Can you work these out from the model? Positions are in its coordinate system, mm. A direction names the side the tool comes from. Round coordinates to 2 decimals unless told otherwise and drop trailing zeros. Loops run counter-clockwise (first coordinate to the right, second up) from the corner with the lowest first, then second, coordinate; pieces in that order, holes last. Notation, with made-up numbers: (-30.75, 80.5) - (-20.75, 80.5) arc R15 cw to (-20.75, 92.5) - close; hole circle Ø2 at (-29, 68). An arc over 180 degrees is marked (long way). Answer as CSV lines item,"result".
```python
from build123d import *

# Parameters (mm, degrees)
F0_W     = 25.4
F0_H     = 5.5252907636
F0_H_2   = 3.9997092364
F0_H_3   = 19.05
F1_DEPTH = 63.5


with BuildPart() as f1:
    # F0 (on Front) → F1 (new body, symmetric)
    with BuildSketch(Plane.XZ):
        with BuildLine():
            ThreePointArc((57.15, 62.6752907636), (56.5270735546, 62.6697350267), (55.9043452947, 62.6530695835))
            add(Edge.make_bspline(
                [(55.9043452947, 62.6530695835), (56.3224009601, 62.6625285107), (56.7376574323, 62.6699360436), (57.15, 62.6752907636)],
                knots=[110.6508010744, 110.6508010744, 110.6508010744, 110.6508010744, 111.8589917407, 111.8589917407, 111.8589917407, 111.8589917407], degree=3))
        make_face()
        with BuildLine():
            add(Edge.make_bspline(
                [(-41.275, 9.525), (-44.1485205161, 43.7142056375), (17.617181224, 61.7867842379), (55.9043452947, 62.6530695835)],
                knots=[0, 0, 0, 0, 110.6508010744, 110.6508010744, 110.6508010744, 110.6508010744], degree=3))
            Line((-41.275, 9.525), (22.225, 9.525))
            Line((22.225, 9.525), (22.225, 27.7502907636))
            ThreePointArc((22.225, 27.7502907636), (32.0177486525, 52.0015910835), (55.9043452947, 62.6530695835))
        make_face()
        with Locations((73.025, 40.8626453818)):
            Rectangle(F0_W, F0_H)
        with Locations((73.025, 64.6751453818)):
            Rectangle(F0_W, F0_H_2)
        Polygon((85.725, 66.675), (85.725, 62.6752907636), (85.725, 43.6252907636), (85.725, 38.1), (111.125, 38.1), (111.125, 66.675), align=None)
        with BuildLine():
            Line((22.225, 27.7502907636), (22.225, 9.525))
            Line((22.225, 9.525), (41.275, 9.525))
            Line((41.275, 9.525), (41.275, 27.7502907636))
            ThreePointArc((41.275, 27.7502907636), (45.9246798487, 38.9756109149), (57.15, 43.6252907636))
            Line((57.15, 43.6252907636), (60.325, 43.6252907636))
            Line((60.325, 43.6252907636), (60.325, 62.6752907636))
            Line((60.325, 62.6752907636), (57.15, 62.6752907636))
            add(Edge.make_bspline(
                [(55.9043452947, 62.6530695835), (56.3224009601, 62.6625285107), (56.7376574323, 62.6699360436), (57.15, 62.6752907636)],
                knots=[110.6508010744, 110.6508010744, 110.6508010744, 110.6508010744, 111.8589917407, 111.8589917407, 111.8589917407, 111.8589917407], degree=3))
            ThreePointArc((55.9043452947, 62.6530695835), (32.0177486525, 52.0015910835), (22.225, 27.7502907636))
        make_face()
        with Locations((73.025, 53.1502907636)):
            Rectangle(F0_W, F0_H_3)
    extrude(amount=F1_DEPTH, both=True)


solid = f1.part
```
Q1. Imagine slicing it at A-A (x = 83). Write out the boundary of the cut face in (y, z) (3 decimals), then the cut area to 3 significant figures.
Checks:
outline,"(-63.5, 38.1) - (63.5, 38.1) - (63.5, 66.675) - (-63.5, 66.675) - close"
area,"3,630 mm²"
Q2. We'd pull the mould along X, two halves only. Please class faces 6 (the flat face through (111.125, -1, 52)), 7 (the flat face through (59, -1, 43.625)), 8 (the flat face through (85, -1, 38.1)): pulls with the +X half, pulls with the -X half, needs draft (parallel to the pull), parting line crosses it, or undercut.
Checks:
face 6,"pulls with the +X half"
face 7,"undercut"
face 8,"needs draft"
Q3. If I drill on line 1 along Z through (x, y) = (103, 13) (3 decimals); line 2 along Z through (x, y) = (28.5, 58) (3 decimals); line 3 along X through (y, z) = (3.5, 29), over which ranges is the centre line in solid material (lowest first)? Write a range as [from, to].
Checks:
line 1,"[38.1, 66.675]"
line 2,"[9.525, 59.658]"
line 3,"[-35.29, 41.32]"
Q4. I'm going to push flat-ended pins straight in: pin 1 Ø3 at (y, z) = (33.5, 31) entering from +X; pin 2 Ø3 at (x, y) = (2.5, 37.5) entering from +Z; pin 3 Ø1.7 at (y, z) = (-19.5, 40.5) entering from -X. Where does each tip first touch, or does it pass through?
Checks:
pin 1,"x = 42"
pin 2,"z = 53.31"
pin 3,"x = -24.04"
Q5. On a 3-axis mill with a long thin cutter (end or side, diameter ignored), from which of +Z, -Z, +X, -X, +Y, -Y can I reach the whole of each face in a straight line? I mean faces 1 (the flat face through (59, -1, 62.675)), 2 (the cylindrical face through (45.8, -0.89, 38.85)), 3 (the flat face through (41.275, -1, 19)), 4 (the flat face through (86, -1, 66.675)), 5 (the flat face through (32, 63.5, 39)). Say none if no direction works.
Checks:
face 1,"+Z, -X, +Y, -Y"
face 2,"-Z, +Y, -Y"
face 3,"-Z, +X, +Y, -Y"
face 4,"+Z, +X, -X, +Y, -Y"
face 5,"+Z, -Z, +X, -X, +Y"
